```python
from build123d import *

# Parameters (mm, degrees)
EXTRUDE_2_DEPTH     = 15
SKETCH_5_R          = 1.25
CUT_EXTRUDE_1_DEPTH = 15


with BuildPart() as part:
    # Эскиз3 → Бобышка-Вытянуть2 (new body)
    with BuildSketch(Plane.XY):
        with BuildLine():
            Line((-1, 12.556672608), (0, 12.556672608))
            Line((0, 12.556672608), (1, 12.556672608))
            Line((1, 12.556672608), (1.403768611, 8.737959355))
            ThreePointArc((1.403768611, 8.737959355), (2.882480289, 8.367425374), (4.275666751, 7.748623996))
            Line((4.275666751, 7.748623996), (6.938281237, 10.513338217))
            Line((6.938281237, 10.513338217), (8.514814211, 9.282670194))
            Line((8.514814211, 9.282670194), (6.483307331, 6.024053955))
            ThreePointArc((6.483307331, 6.024053955), (7.419229042, 4.824680344), (8.135910959, 3.482736406))
            Line((8.135910959, 3.482736406), (11.938429132, 4.017951822))
            Line((11.938429132, 4.017951822), (12.423885361, 2.077763107))
            Line((12.423885361, 2.077763107), (8.823580607, 0.683319303))
            ThreePointArc((8.823580607, 0.683319303), (8.813761391, -0.800068834), (8.556312106, -2.260978362))
            Line((8.556312106, -2.260978362), (11.88304599, -4.178904758))
            Line((11.88304599, -4.178904758), (11.071850771, -6.007008197))
            Line((11.071850771, -6.007008197), (7.417581711, -4.827212608))
            ThreePointArc((7.417581711, -4.827212608), (6.479864305, -6.027757343), (5.350154649, -7.049705329))
            Line((5.350154649, -7.049705329), (6.785807353, -10.588258594))
            Line((6.785807353, -10.588258594), (5.913418577, -11.077071262))
            Line((5.913418577, -11.077071262), (5.041029802, -11.565883931))
            Line((5.041029802, -11.565883931), (2.88053291, -8.36809597))
            ThreePointArc((2.88053291, -8.36809597), (0.000835422, -8.849999961), (-2.878952996, -8.368639653))
            Line((-2.878952996, -8.368639653), (-5.029072142, -11.548959277))
            Line((-5.029072142, -11.548959277), (-5.911327166, -11.078187493))
            Line((-5.911327166, -11.078187493), (-6.783800352, -10.589525504))
            Line((-6.783800352, -10.589525504), (-5.348823599, -7.050715291))
            ThreePointArc((-5.348823599, -7.050715291), (-6.479295244, -6.028369028), (-7.417581672, -4.827212668))
            Line((-7.417581672, -4.827212668), (-11.071850724, -6.007008285))
            Line((-11.071850724, -6.007008285), (-11.883045968, -4.178904821))
            Line((-11.883045968, -4.178904821), (-8.556312093, -2.260978407))
            ThreePointArc((-8.556312093, -2.260978407), (-8.817386806, -0.759071749), (-8.816843455, 0.765357101))
            Line((-8.816843455, 0.765357101), (-12.423885379, 2.077762999))
            Line((-12.423885379, 2.077762999), (-11.938429167, 4.017951718))
            Line((-11.938429167, 4.017951718), (-8.138356697, 3.477017439))
            ThreePointArc((-8.138356697, 3.477017439), (-7.419229073, 4.824680297), (-6.479071962, 6.028609003))
            Line((-6.479071962, 6.028609003), (-8.514814242, 9.282670165))
            Line((-8.514814242, 9.282670165), (-6.938281272, 10.513338193))
            Line((-6.938281272, 10.513338193), (-4.275666751, 7.748623996))
            ThreePointArc((-4.275666751, 7.748623996), (-2.882480289, 8.367425373), (-1.403768611, 8.737959355))
            Line((-1.403768611, 8.737959355), (-1, 12.556672608))
        make_face()
    extrude(amount=EXTRUDE_2_DEPTH)

    # Эскиз5 → Вырез-Вытянуть1 (cut)
    with BuildSketch(Plane(origin=(0, 0, 0), x_dir=(-1, 0, 0), z_dir=(0, 0, -1))):
        Circle(SKETCH_5_R)
    extrude(amount=-CUT_EXTRUDE_1_DEPTH, mode=Mode.SUBTRACT)


solid = part.part
```
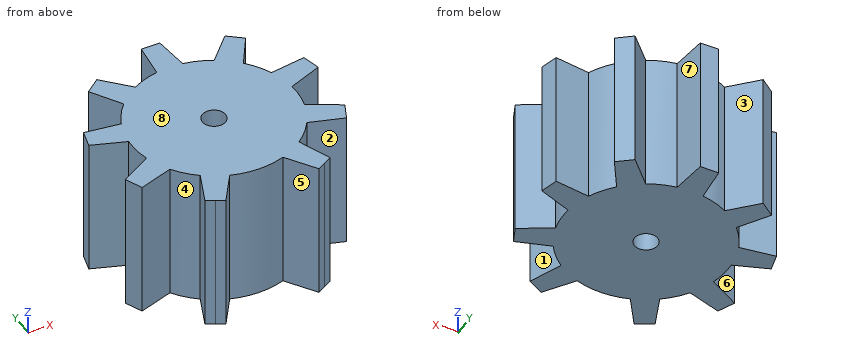
Geometry check sheet. Reference: the model listing, model coordinates, mm. Face numbers are marked on the shaded views. A direction names the side the tool comes from. Round coordinates to 2 decimals unless told otherwise and drop trailing zeros. Loops run counter-clockwise (first coordinate to the right, second up) from the corner with the lowest first, then second, coordinate; pieces in that order, holes last. Notation, with made-up numbers: (25.25, 37) -> (54.25, 37) arc R14 ccw to (54.25, 51) -> close; hole circle Ø8 at (-9, 85.5). An arc over 180 degrees is marked (long way). Use a Markdown table: item, result.
(1) Sectioned sample at A-A (y = 0). Enter the section's corners in (x, z), then the cut area to 3 significant figures.
Calculated:
| item | result |
|---|---|
| outline | (-8.85, 0) -> (-1.25, 0) -> (-1.25, 15) -> (-8.85, 15) -> close; (1.25, 0) -> (8.85, 0) -> (8.85, 15) -> (1.25, 15) -> close |
| area | 228 mm² |
(2) Go/stop test with flat-tipped pins: P1, Ø1, axis at y = -1, z = 7, coming from the +X side; P2, Ø5, axis at y = 9, z = 13, coming from the -X side; P3, Ø6, axis at y = 6, z = 10.5, coming from the -X side. Record where each tip stops, or that it passes through.
Calculated:
| item | result |
|---|---|
| P1 | x = 8.84 |
| P2 | x = -8.51 |
| P3 | x = -12.19 |
(3) Scan lines: probe 1 along Y at (x, z) = (0, 8); probe 2 along Y at (x, z) = (-10.5, 9.5); probe 3 along X at (y, z) = (-0.5, 1.5). Record each from-to range of solid material in increasing order.
Calculated:
| item | result |
|---|---|
| probe 1 | -8.85 to -1.25, 1.25 to 12.56 |
| probe 2 | -5.82 to -3.38, 1.38 to 3.81 |
| probe 3 | -8.84 to -1.15, 1.15 to 8.84 |
(4) Mould release check, pull along Y, two halves, no side actions. Record for the marked faces 5, 6, 7 and 8: released by +Y, released by -Y, zero draft, split by the parting line, or undercut.
Calculated:
| item | result |
|---|---|
| face 5 | released by -Y |
| face 6 | undercut |
| face 7 | released by +Y |
| face 8 | zero draft |
(5) Set-up check for the marked faces 1, 2, 3 and 4: record each of +Z, -Z, +X, -X, +Y, -Y from which the full face is reachable in a straight line by a thin tool's end or side.
Calculated:
| item | result |
|---|---|
| face 1 | +Z, -Z, +X |
| face 2 | +Z, -Z, -Y |
| face 3 | +Z, -Z, +Y |
| face 4 | +Z, -Z |
(6) Sectioned sample at C-C (y = 5.5). Enter the section's corners in (x, z), then the cut area to 3 significant figures.
Calculated:
| item | result |
|---|---|
| outline | (-6.93, 0) -> (6.93, 0) -> (6.93, 15) -> (-6.93, 15) -> close |
| area | 208 mm² |
(7) Sectioned sample at B-B (x = 0). Enter the section's corners in (y, z).
Calculated:
| item | result |
|---|---|
| outline | (-8.85, 0) -> (-1.25, 0) -> (-1.25, 15) -> (-8.85, 15) -> close; (1.25, 0) -> (12.56, 0) -> (12.56, 15) -> (1.25, 15) -> close |
